Drawing for the job (mm, zero at the part's lowest x, y, z). A direction names the side the tool comes from. Round coordinates to 2 decimals unless told otherwise and drop trailing zeros. Loops run counter-clockwise (first coordinate to the right, second up) from the corner with the lowest first, then second, coordinate; pieces in that order, holes last. Notation, with made-up numbers: M 57,45.5 L 95,45.5 A21 ccw 95,77.5 Z; hole C 63,63.5 d5. An arc over 180 degrees is marked long. Use a Markdown table: item, result. Add a question column.
Q1. Pin check, flat tip, straight feed: pin 1 (1 mm diameter, centred on x = 2, z = 7, fed in from +Y). Stop position of the tip, or through.
Q2. Tool access for the marked faces 1 and 2: list every direction of +Z, -Z, +X, -X, +Y, -Y with a clear straight run to the whole face (end or side of a thin tool).
Q3. Probe line 1 (Y direction, x = 2.25, z = 2.5); line 2 (X direction, y = 2.85, z = 6) (1 decimal); line 3 (Y direction, x = 2.75, z = 6.75) (1 decimal). List the from-to ranges inside material, lowest first. Write a range as from..to.
Q4. Cut at D-D (y = 4.1). Give the cut face in (x, z).
Q5. Cut at C-C (z = 6.25). Give the cut face in (x, y).
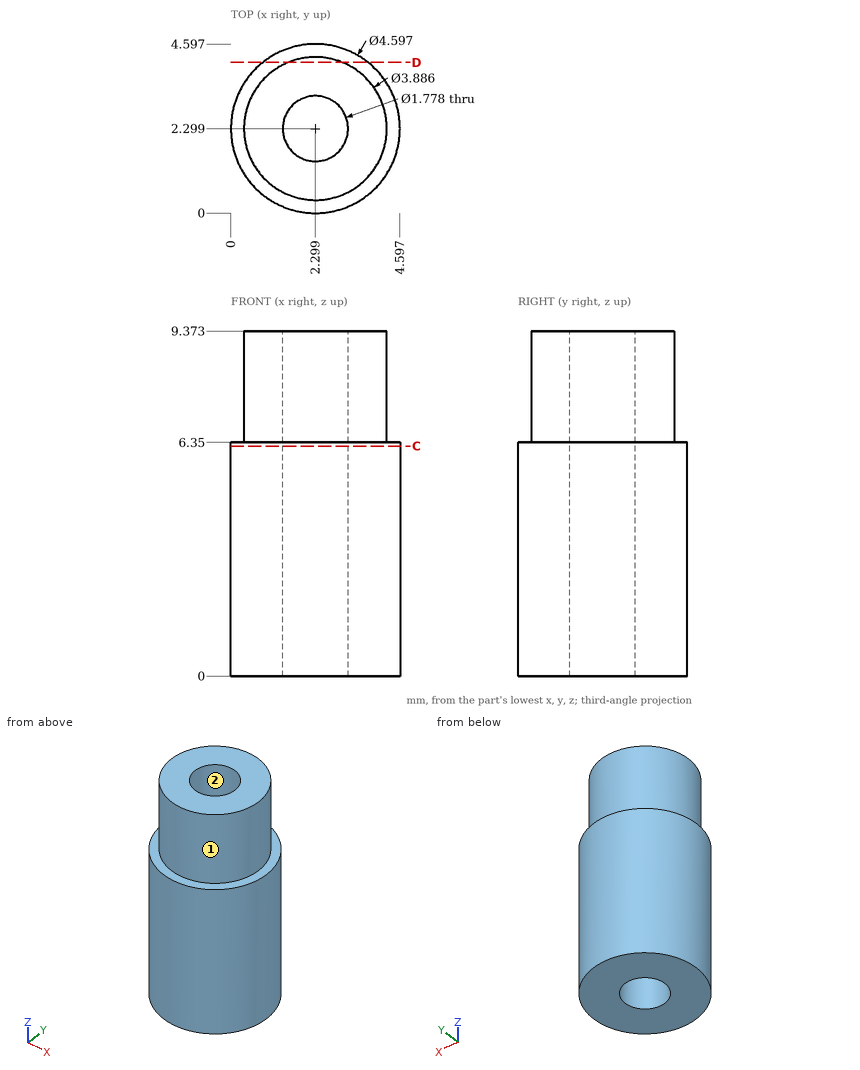
Checked values:
| question | item | result |
|---|---|---|
| 1 | pin 1 | stops at y = 4.24 |
| 2 | face 1 | +Z |
| 2 | face 2 | +Z, -Z |
| 3 | line 1 | y = 0..1.41, 3.19..4.6 |
| 3 | line 2 | x = 0.1..1.6, 3..4.5 |
| 3 | line 3 | y = 0.4..1.5, 3.1..4.2 |
| 4 | outline | M 0.87,0 L 3.73,0 L 3.73,6.35 L 3.03,6.35 L 3.03,9.37 L 1.57,9.37 L 1.57,6.35 L 0.87,6.35 Z |
| 5 | outline | C 2.3,2.3 d4.6; hole C 2.3,2.3 d1.78 |
